Source: CAD feature listing. Evaluate the final solid. Frame: model axes, mm. A direction names the side the tool comes from. Round coordinates to 2 decimals unless told otherwise and drop trailing zeros. Loops run counter-clockwise (first coordinate to the right, second up) from the corner with the lowest first, then second, coordinate; pieces in that order, holes last. Notation, with made-up numbers: (7, -38) - (65, -38) arc R14 cw to (65, -32) - close; hole circle Ø9 at (-31, -25.5). An arc over 180 degrees is marked (long way). One line per question, with ' | ' between items.
from build123d import *

# Parameters (mm, degrees)
ESQUISSE1_W             = 40
ESQUISSE1_H             = 20
BOSS_EXTRU_2_DEPTH      = 14.1
ESQUISSE2_W             = 2.5
ESQUISSE2_H             = 2.5
ENL_V_MAT_EXTRU_1_DEPTH = 27.435014659


with BuildPart() as part:
    # Esquisse1 → Boss.-Extru.2 (new body)
    with BuildSketch(Plane(origin=(0, 0, 0), x_dir=(1, 0, 0), z_dir=(0, 1, 0))):
        Rectangle(ESQUISSE1_W, ESQUISSE1_H)
    extrude(amount=BOSS_EXTRU_2_DEPTH)

    # Esquisse2 → Enlèv. mat.-Extru.1 (cut, through all)
    with BuildSketch(Plane(origin=(0, 14.1, 0), x_dir=(1, 0, 0), z_dir=(0, 1, 0))):
        with Locations((-2.9, 0)):
            Rectangle(ESQUISSE2_W, ESQUISSE2_H)
        Rectangle(ESQUISSE2_W, ESQUISSE2_H)
        with Locations((2.9, 0)):
            Rectangle(ESQUISSE2_W, ESQUISSE2_H)
    extrude(amount=-ENL_V_MAT_EXTRU_1_DEPTH, mode=Mode.SUBTRACT)


solid = part.part
1. Mould query, pull axis X, two halves, no side actions, for faces 1 (the flat face through (-20, 7, 0)), 2 (the flat face through (0, 0, -2)), 3 (the flat face through (0, 7, -1.25)). Classes: released by +X, released by -X, zero draft, split by the parting line, or undercut.
Worked out:
face 1: released by -X | face 2: zero draft | face 3: undercut
2. Access query for faces 4 (the flat face through (3, 7, -1.25)), 5 (the flat face through (0, 7, -10)). Directions: +Z, -Z, +X, -X, +Y, -Y. A direction counts if a zero-diameter tool reaches every point of the face in a straight line with its end or side. Return the directions, or none.
Worked out:
face 4: +Y, -Y | face 5: -Z, +X, -X, +Y, -Y
3. Section query B-B, the plane y = 7.5. Return loops of the section in (x, z).
Worked out:
outline: (-20, -10) - (20, -10) - (20, 10) - (-20, 10) - close; hole (-4.15, -1.25) - (-1.65, -1.25) - (-1.65, 1.25) - (-4.15, 1.25) - close; hole (-1.25, -1.25) - (1.25, -1.25) - (1.25, 1.25) - (-1.25, 1.25) - close; hole (1.65, -1.25) - (4.15, -1.25) - (4.15, 1.25) - (1.65, 1.25) - close
4. Section query A-A, the plane z = 0. Return loops of the section in (x, y).
Worked out:
outline: (-20, 0) - (-4.15, 0) - (-4.15, 14.1) - (-20, 14.1) - close; (-1.65, 0) - (-1.25, 0) - (-1.25, 14.1) - (-1.65, 14.1) - close; (1.25, 0) - (1.65, 0) - (1.65, 14.1) - (1.25, 14.1) - close; (4.15, 0) - (20, 0) - (20, 14.1) - (4.15, 14.1) - close
5. Material intervals for probe 1 along X at (y, z) = (6, 0.25); probe 2 along Z at (x, y) = (-4, 6.25), sorted ascending.
Worked out:
probe 1: x = -20 to -4.15, -1.65 to -1.25, 1.25 to 1.65, 4.15 to 20 | probe 2: z = -10 to -1.25, 1.25 to 10
